For this review, take the finished solid that the model builds, in its own axes (mm). Face numbers are marked on the shaded views. A direction names the side the tool comes from. Round coordinates to 2 decimals unless told otherwise and drop trailing zeros. Write each loop counter-clockwise with the first axis right and the second up, starting at its lowest first coordinate (ties: lowest second). Pieces come first, ordered by that corner, then holes. Notation, with made-up numbers: (-7, -10.5) -> (42, -10.5) arc R36 cw to (42, 27.5) -> close; hole circle Ø2 at (-19.5, 12). An arc over 180 degrees is marked (long way). Answer as CSV lines item,"result". Start each with the question number.
Item 1: Wall thickness on probe 1 along Y at (x, z) = (-3.5, 3.25); probe 2 along Z at (x, y) = (0, 9.4); probe 3 along X at (y, z) = (-8, 9.25): over which ranges is each line inside the solid? List them lowest first. Write a range as from..to.
Item 2: For pin 1 Ø3.5 at (x, y) = (-6.45, -6.45) entering from -Z; pin 2 Ø2.5 at (x, y) = (-20, 7.5) entering from -Z, all flat-tipped, find the tip position at first contact; note any pin that passes through.
Item 3: Take a section at D-D on z = 9.25. Give the boundary of the cut face in (x, y).
Item 4: Take a section at C-C on y = 8. Give the boundary of the cut face in (x, z).
Item 5: Take a section at B-B on x = 20. Give the boundary of the cut face in (y, z).
Item 6: Take a section at A-A on x = -20. Give the boundary of the cut face in (y, z).
Item 7: Machinability: for the marked faces 1 and 2, which of the approach directions +Z, -Z, +X, -X, +Y, -Y give a long, thin tool a straight path to every point of the face, cutting with its end or side? Answer none if there is none.
Item 8: Mouldability with a two-part tool opening along Y and no side actions: class the marked faces 3, 4, 5 and 6 as +Y half, -Y half, draft (parallel to the pull), parting line (faces both ways), or undercut.
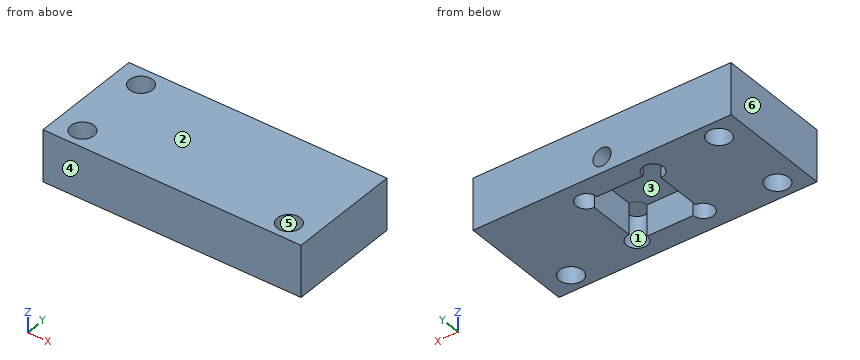
```python
from build123d import *

# Parameters (mm, degrees)
SKIZZE1_W                       = 50
SKIZZE1_H                       = 22
AUFSATZ_LINEAR_AUSTRAGEN1_DEPTH = 10
SKIZZE2_R                       = 2.25
SCHNITT_LINEAR_AUSTRAGEN1_DEPTH = 11
SKIZZE3_W                       = 12.9
SKIZZE3_H                       = 12.9
SCHNITT_LINEAR_AUSTRAGEN2_DEPTH = 6
SKIZZE4_R                       = 2
SCHNITT_LINEAR_AUSTRAGEN3_DEPTH = 6.1
SKIZZE5_R                       = 1.75
SCHNITT_LINEAR_AUSTRAGEN4_DEPTH = 6.1


with BuildPart() as part:
    # Skizze1 → Aufsatz-Linear austragen1 (new body)
    with BuildSketch(Plane.XY):
        Rectangle(SKIZZE1_W, SKIZZE1_H)
    extrude(amount=AUFSATZ_LINEAR_AUSTRAGEN1_DEPTH)

    # Skizze2 → Schnitt-Linear austragen1 (cut, through all)
    with BuildSketch(Plane.XY.offset(10)):
        with Locations((-20, 7.5)):
            Circle(SKIZZE2_R)
        with Locations((-20, -7.5)):
            Circle(SKIZZE2_R)
        with Locations((20, -7.5)):
            Circle(SKIZZE2_R)
    extrude(amount=-SCHNITT_LINEAR_AUSTRAGEN1_DEPTH, mode=Mode.SUBTRACT)

    # Skizze3 → Schnitt-Linear austragen2 (cut)
    with BuildSketch(Plane(origin=(0, 0, 0), x_dir=(-1, 0, 0), z_dir=(0, 0, -1))):
        Rectangle(SKIZZE3_W, SKIZZE3_H)
    extrude(amount=-SCHNITT_LINEAR_AUSTRAGEN2_DEPTH, mode=Mode.SUBTRACT)

    # Skizze4 → Schnitt-Linear austragen3 (cut)
    with BuildSketch(Plane(origin=(0, 0, 0), x_dir=(-1, 0, 0), z_dir=(0, 0, -1))):
        with Locations((-6.45, 6.45)):
            Circle(SKIZZE4_R)
        with Locations((6.45, 6.45)):
            Circle(SKIZZE4_R)
        with Locations((-6.45, -6.45)):
            Circle(SKIZZE4_R)
        with Locations((6.45, -6.45)):
            Circle(SKIZZE4_R)
    extrude(amount=-SCHNITT_LINEAR_AUSTRAGEN3_DEPTH, mode=Mode.SUBTRACT)

    # Skizze5 → Schnitt-Linear austragen4 (cut)
    with BuildSketch(Plane(origin=(0, 11, 0), x_dir=(1, 0, 0), z_dir=(0, 1, 0))):
        with Locations((0, -3)):
            Circle(SKIZZE5_R)
    extrude(amount=-SCHNITT_LINEAR_AUSTRAGEN4_DEPTH, mode=Mode.SUBTRACT)


solid = part.part
```
Output values:
1,probe 1,"y = -11..-6.45, 6.45..11"
1,probe 2,"z = 0..1.25, 4.75..10"
1,probe 3,"x = -25..-22.19, -17.81..17.81, 22.19..25"
2,pin 1,"stops at z = 6.1"
2,pin 2,"passes through"
3,outline,"(-25, -11) -> (25, -11) -> (25, 11) -> (-25, 11) -> close; hole circle Ø4.5 at (-20, -7.5); hole circle Ø4.5 at (-20, 7.5); hole circle Ø4.5 at (20, -7.5)"
4,outline,"(-25, 0) -> (-22.19, 0) -> (-22.19, 10) -> (-25, 10) -> close; (-17.81, 0) -> (-7.71, 0) -> (-7.71, 6.1) -> (-5.19, 6.1) -> (-5.19, 0) -> (5.19, 0) -> (5.19, 6.1) -> (7.71, 6.1) -> (7.71, 0) -> (25, 0) -> (25, 10) -> (-17.81, 10) -> close; hole circle Ø3.5 at (0, 3)"
5,outline,"(-11, 0) -> (-9.75, 0) -> (-9.75, 10) -> (-11, 10) -> close; (-5.25, 0) -> (11, 0) -> (11, 10) -> (-5.25, 10) -> close"
6,outline,"(-11, 0) -> (-9.75, 0) -> (-9.75, 10) -> (-11, 10) -> close; (-5.25, 0) -> (5.25, 0) -> (5.25, 10) -> (-5.25, 10) -> close; (9.75, 0) -> (11, 0) -> (11, 10) -> (9.75, 10) -> close"
7,face 1,"-Z"
7,face 2,"+Z, +X, -X, +Y, -Y"
8,face 3,"undercut"
8,face 4,"-Y half"
8,face 5,"undercut"
8,face 6,"draft"
